Design review of the part built by this model. Coordinates are the model's own, in mm. Give positions to 0.01 mm unless a question says otherwise; leave off trailing zeros. Order: outer loops, then holes, each group sorted by start corner. A loop starts at its lowest first (then second) coordinate and runs counter-clockwise, first axis right, second up. Notation, with made-up numbers: M -24,18.25 L -15,18.25 A6 ccw -15,23.25 Z; hole C -21.75,42.5 d10. An arc over 180 degrees is marked long. Answer as a JSON object with one key per item and string values.
from build123d import *

# Parameters (mm, degrees)
SKETCH_1_W      = 15.4
SKETCH_1_H      = 3
SKETCH_1_R      = 0.6
EXTRUDE_1_DEPTH = 1.6
FILLET_1_R      = 1.5


with BuildPart() as part:
    # 草图1 → 凸台-拉伸1 (new body)
    with BuildSketch(Plane(origin=(0, 0, 0), x_dir=(0, 0, -1), z_dir=(1, 0, 0))):
        with Locations((7.7, -1.5)):
            Rectangle(SKETCH_1_W, SKETCH_1_H)
        with Locations((1.5, -1.5)):
            Circle(SKETCH_1_R, mode=Mode.SUBTRACT)
        with Locations((14, -1.5)):
            Circle(SKETCH_1_R, mode=Mode.SUBTRACT)
    extrude(amount=EXTRUDE_1_DEPTH)

    # 圆角1
    fillet_1_edges = [part.edges().sort_by_distance(p)[0] for p in [
        (0.8, -3, 0),
        (0.8, 0, 0),
        (0.8, -3, -15.4),
        (0.8, 0, -15.4),
    ]]
    fillet(fillet_1_edges, radius=FILLET_1_R - 0.0001)  # a hair under: the kernel refuses the full size


solid = part.part
(1) We need section C-C (y = -2.6). Write out the cut boundary in (x, z).
Checked values:
{"outline": "M 0,-14.92 L 1.6,-14.92 L 1.6,-0.48 L 0,-0.48 Z"}
(2) We need section B-B (y = -0.65). Write out the cut boundary in (x, z).
Checked values:
{"outline": "M 0,-15.14 L 1.6,-15.14 L 1.6,-0.26 L 0,-0.26 Z"}
(3) Draft analysis for pull direction Y (two halves, no side actions). For faces 1 (the flat face through (0, -1, -8)), 2 (the cylindrical face through (0.81, -2.57, -14.95)), 3 (the flat face through (1, 0, -8)), 4 (the cylindrical face through (0.789, -1.32, -14.572)), state which applies: +Y half, -Y half, draft (parallel to the pull), parting line (faces both ways), or undercut.
Checked values:
{"face 1": "draft", "face 2": "-Y half", "face 3": "+Y half", "face 4": "undercut"}
(4) To check wall thickness, follow L1, parallel to Z at x = 0.55, y = -1.4; L2, parallel to Y at x = 1.15, z = -14; L3, parallel to Z at x = 0.35, y = -1.9. State the ranges of each line that lie inside material, in increasing order. Write a range as from..to.
Checked values:
{"L1": "z = -15.4..-14.59, -13.41..-2.09, -0.91..0", "L2": "y = -3..-2.1, -0.9..0", "L3": "z = -15.35..-14.45, -13.55..-1.95, -1.05..-0.05"}
(5) We need section A-A (x = 1.2). Count the separate pieces of the cut face and the enclosed holes in it, plus the area to 3 significant figures.
Checked values:
{"separate pieces": "1", "enclosed holes": "2", "area": "42.0 mm^2"}
